Verification items for the finished model (mm, model axes). Coordinates: 2 decimals unless noted, no trailing zeros. Order: outer loops, then holes, each group sorted by start corner. A loop starts at its lowest first (then second) coordinate and runs counter-clockwise, first axis right, second up. Notation, with made-up numbers: (-2.75, 46) -> (27.25, 46) arc R14 cw to (27.25, 67) -> close; hole circle Ø10 at (-21, -22.5). An arc over 180 degrees is marked (long way). Use CSV: the item, a comma, the result in double quotes. Start each with the question number.
1) Scan lines: line 1 along Y through (x, z) = (13.5, -3); line 2 along Y through (x, z) = (25, -1.5); line 3 along X through (y, z) = (-63, -1.5). Record each from-to range of solid material in increasing order.
2) Sectioned sample at C-C on x = -256. Record the boundary of the cut face in (y, z) (3 decimals), then the cut area to 3 significant figures.
3) Sectioned sample at D-D on y = 195. Record the boundary of the cut face in (x, z) (3 decimals).
4) Release check for a two-part mould opening along X. For faces 1 (the flat face through (-256.284, 115.577, 0.044)), 2 (the flat face through (-113, 106, -3.175)), 3 (the cylindrical face through (79.14, -61.13, 0.04)) record: released by +X, released by -X, zero draft, split by the parting line, or undercut.
5) Go/stop test with flat-tipped pins: pin 1 (1 mm diameter, centred on y = 189, z = 2.5, fed in from +X); pin 2 (6.5 mm diameter, centred on x = 15, y = 0, fed in from +Z) (3 decimals); pin 3 (0.8 mm diameter, centred on y = 304, z = -1, fed in from -X); pin 4 (0.8 mm diameter, centred on y = 304, z = 1.5, fed in from +X). Record where each tip stops, or that it passes through.
6) Sectioned sample at B-B on z = 0.5. Give the number of separate pieces and of enclosed holes in the cut face, then the cut area to 3 significant figures.
7) Sectioned sample at A-A on x = 29. Record the boundary of the cut face in (y, z) (3 decimals).
from build123d import *

# Parameters (mm, degrees)
SKETCH1_W           = 6.35
SKETCH1_H           = 65
SKETCH1_W_2         = 65
SKETCH1_H_2         = 6.35
BOSS_EXTRUDE1_DEPTH = 3.175
SKETCH2_W           = 50
SKETCH2_H           = 6.35
BOSS_EXTRUDE2_DEPTH = 6.35
SKETCH3_R           = 2
CUT_EXTRUDE1_DEPTH  = 7.35
FILLET1_R           = 1
SKETCH4_R           = 2
CUT_EXTRUDE2_DEPTH  = 7.35
FILLET2_R           = 1
FILLET3_R           = 2


with BuildPart() as part:
    # Sketch1 → Boss-Extrude1 (new body, symmetric)
    with BuildSketch(Plane.XY):
        with BuildLine():
            Line((-360, 300), (-440, 300))
            Line((-440, 300), (-70.846389974, -70.574705296))
            ThreePointArc((-70.846389974, -70.574705296), (80.595787705, -59.197288825), (46.150399684, 88.713812955))
            Line((46.150399684, 88.713812955), (-360, 300))
        make_face()
        with Locations((-3.175, -47.5)):
            Rectangle(SKETCH1_W, SKETCH1_H, mode=Mode.SUBTRACT)
        with Locations((47.5, 3.175)):
            Rectangle(SKETCH1_W_2, SKETCH1_H_2, mode=Mode.SUBTRACT)
    extrude(amount=BOSS_EXTRUDE1_DEPTH, both=True)

    # Sketch2 → Boss-Extrude2 (add)
    with BuildSketch(Plane.XY.offset(3.175)):
        with Locations((-400, 303.175)):
            Rectangle(SKETCH2_W, SKETCH2_H)
    extrude(amount=-BOSS_EXTRUDE2_DEPTH)

    # Sketch3 → Cut-Extrude1 (cut, through all)
    with BuildSketch(Plane.XY.offset(3.175)):
        with Locations((-6.35, -15)):
            Circle(SKETCH3_R)
        with Locations((0, -15)):
            Circle(SKETCH3_R)
        with Locations((-6.35, -80)):
            Circle(SKETCH3_R)
        with Locations((0, -80)):
            Circle(SKETCH3_R)
        with Locations((15, 0)):
            Circle(SKETCH3_R)
        with Locations((15, 6.35)):
            Circle(SKETCH3_R)
        with Locations((80, 6.35)):
            Circle(SKETCH3_R)
        with Locations((80, 0)):
            Circle(SKETCH3_R)
    extrude(amount=-CUT_EXTRUDE1_DEPTH, mode=Mode.SUBTRACT)

    # Fillet1
    fillet1_edges = [part.edges().sort_by_distance(p)[0] for p in [
        (17, 6.35, 0),
        (80, 4.35, 0),
        (78, 0, 0),
        (-6.35, -17, 0),
        (15, 4.35, 0),
        (15, 2, 0),
        (78, 6.35, 0),
        (80, 2, 0),
        (-4.35, -15, 0),
        (-2, -15, 0),
        (0, -78, 0),
        (-4.35, -80, 0),
        (17, 0, 0),
        (-2, -80, 0),
        (-6.35, -78, 0),
        (0, -17, 0),
    ]]
    fillet(fillet1_edges, radius=FILLET1_R)

    # Sketch4 → Cut-Extrude2 (cut, through all)
    with BuildSketch(Plane.XY.offset(3.175)):
        with Locations((-425, 300)):
            Circle(SKETCH4_R)
        with Locations((-375, 300)):
            Circle(SKETCH4_R)
    extrude(amount=-CUT_EXTRUDE2_DEPTH, mode=Mode.SUBTRACT)

    # Fillet2
    fillet2_edges = [part.edges().sort_by_distance(p)[0] for p in [
        (-375, 302, 0),
        (-425, 302, 0),
        (-427, 300, 0),
        (-373, 300, 0),
        (-425, 306.35, 0),
        (-375, 306.35, 0),
    ]]
    fillet(fillet2_edges, radius=FILLET2_R)

    # Fillet3
    fillet3_edges = [part.edges().sort_by_distance(p)[0] for p in [
        (-440, 300, 0),
        (-360, 300, 0),
    ]]
    fillet(fillet3_edges, radius=FILLET3_R)


solid = part.part
Answers follow:
1,line 1,"y = -99.08 to -1.32, 1.32 to 5.03, 7.67 to 105.7"
1,line 2,"y = -96.82 to 0, 6.35 to 99.72"
1,line 3,"x = -78.39 to -6.35, 0 to 77.66"
2,outline,"(115.292, -3.175) -> (245.897, -3.175) -> (245.897, 3.175) -> (115.292, 3.175) -> close"
2,area,"829 mm²"
3,outline,"(-335.403, -3.175) -> (-158.161, -3.175) -> (-158.161, 3.175) -> (-335.403, 3.175) -> close"
4,face 1,"released by -X"
4,face 2,"zero draft"
4,face 3,"split by the parting line"
5,pin 1,"stops at x = -145.67"
5,pin 2,"stops at z = 3.175"
5,pin 3,"stops at x = -425"
5,pin 4,"stops at x = -375"
6,separate pieces,"1"
6,enclosed holes,"2"
6,area,"77,700 mm²"
7,outline,"(-95.703, -3.175) -> (0, -3.175) -> (0, 3.175) -> (-95.703, 3.175) -> close; (6.35, -3.175) -> (97.636, -3.175) -> (97.636, 3.175) -> (6.35, 3.175) -> close"
